Could you check a few things on this model? Use its own coordinates, in mm. A direction names the side the tool comes from. Coordinates: 2 decimals unless noted, no trailing zeros. Loops run counter-clockwise (first coordinate to the right, second up) from the corner with the lowest first, then second, coordinate; pieces in that order, holes last. Notation, with made-up numbers: (49, 65.5) -> (90, 65.5) arc R30 ccw to (90, 97.5) -> close; hole circle Ø3 at (-37, 52.5). An arc over 180 degrees is marked (long way). One line per question, with ' | ' between items. Start each with the question number.
(1) If we mould it in two halves opening along Z, with no side actions, what happens to faces 6 (the face through (-6.726, 0, 41)), 7 (the face through (-39.738, 0, 70)), 8 (the face through (-67, 0, 0))? For each: pulls with the +Z half, pulls with the -Z half, needs draft (parallel to the pull), parting line crosses it, or undercut.
(2) Which directions (+Z, -Z, +X, -X, +Y, -Y) give clear straight access to the entire face, cutting with the end or side of a thin tool? Please do faces 1 (the face through (0, 0, 0)), 2 (the face through (-72.403, -0.178, 51.609)), 3 (the face through (-4, 0, 34.364)), 4 (the face through (-39.738, 0, 11)), 5 (the face through (-19.77, -0.18, 77.01)).
(3) Suppose I cut it at A-A (x = -5.5). Please give me the cut outline in (y, z), plus the area to 3 significant figures.
(4) If I drill on line 1 along Z through (x, y) = (-61.5, -6.75); line 2 along X through (y, z) = (-6.75, 68); line 3 along X through (y, z) = (-10.75, 41), over which ranges is the centre line in solid material (lowest first)?
(5) Suppose I cut it at D-D (z = 41.5). Please give me the cut outline in (x, y).
(6) Suppose I cut it at C-C (y = 1.25). Please give me the cut outline in (x, z), plus the area to 3 significant figures.
(7) Suppose I cut it at B-B (z = 69.5). Please give me the cut outline in (x, y).
(8) I'm going to push flat-ended pins straight in: pin 1 Ø6.5 at (x, y) = (-32.5, 5) entering from +Z; pin 2 Ø12 at (y, z) = (5.5, 49.5) entering from -X; pin 3 Ø1.5 at (x, y) = (-4.5, -2.5) entering from -Z; pin 4 Ø14 at (y, z) = (2.5, 42) entering from +X. Where does each tip first touch, or does it pass through?
```python
from build123d import *

# Parameters (mm, degrees)
F1_DEPTH = 12.7


with BuildPart() as f1:
    # F0 (on Front) → F1 (new body, symmetric)
    with BuildSketch(Plane.XZ):
        Polygon((-60.049345, 47.064326), (-60.049345, 40.714326), (-6.725921, 40.714326), (-6.725921, 47.064326), (-1.645921, 47.064326), (12.7, 56.028652), (12.7, 81.428652), (-12.7, 81.428652), (-27.037633, 72.469505), (-27.037633, 67.389505), (-39.737633, 67.389505), (-39.737633, 72.469505), (-54.075266, 81.428652), (-79.475266, 81.428652), (-79.475266, 56.028652), (-65.129345, 47.064326), align=None)
        Polygon((-65.129345, 34.364326), (-79.475266, 25.4), (-79.475266, 0), (-54.075266, 0), (-39.737633, 8.959147), (-39.737633, 14.039147), (-27.037633, 14.039147), (-27.037633, 8.959147), (-12.7, 0), (12.7, 0), (12.7, 25.4), (-1.645921, 34.364326), (-6.725921, 34.364326), (-6.725921, 40.714326), (-60.049345, 40.714326), (-60.049345, 34.364326), align=None)
    extrude(amount=F1_DEPTH, both=True)


solid = f1.part
```
Checks:
1) face 6: undercut | face 7: needs draft | face 8: pulls with the -Z half
2) face 1: -Z, +X, -X, +Y, -Y | face 2: -X, +Y, -Y | face 3: +X, +Y, -Y | face 4: -Z, +Y, -Y | face 5: +Z, +Y, -Y
3) outline: (-12.7, 0) -> (12.7, 0) -> (12.7, 34.36) -> (-12.7, 34.36) -> close; (-12.7, 47.06) -> (12.7, 47.06) -> (12.7, 81.43) -> (-12.7, 81.43) -> close | area: 1,750 mm^2
4) line 1: z = 0 to 34.36, 47.06 to 81.43 | line 2: x = -79.48 to -39.74, -27.04 to 12.7 | line 3: x = -60.05 to -6.73
5) outline: (-60.05, -12.7) -> (-6.73, -12.7) -> (-6.73, 12.7) -> (-60.05, 12.7) -> close
6) outline: (-79.48, 0) -> (-54.08, 0) -> (-39.74, 8.96) -> (-39.74, 14.04) -> (-27.04, 14.04) -> (-27.04, 8.96) -> (-12.7, 0) -> (12.7, 0) -> (12.7, 25.4) -> (-1.65, 34.36) -> (-6.73, 34.36) -> (-6.73, 47.06) -> (-1.65, 47.06) -> (12.7, 56.03) -> (12.7, 81.43) -> (-12.7, 81.43) -> (-27.04, 72.47) -> (-27.04, 67.39) -> (-39.74, 67.39) -> (-39.74, 72.47) -> (-54.08, 81.43) -> (-79.48, 81.43) -> (-79.48, 56.03) -> (-65.13, 47.06) -> (-60.05, 47.06) -> (-60.05, 34.36) -> (-65.13, 34.36) -> (-79.48, 25.4) -> close | area: 6,140 mm^2
7) outline: (-79.48, -12.7) -> (-39.74, -12.7) -> (-39.74, 12.7) -> (-79.48, 12.7) -> close; (-27.04, -12.7) -> (12.7, -12.7) -> (12.7, 12.7) -> (-27.04, 12.7) -> close
8) pin 1: stops at z = 67.39 | pin 2: stops at x = -78.63 | pin 3: stops at z = 0 | pin 4: stops at x = 1.45
